Could you check a few things on this model? Use its own coordinates, in mm. A direction names the side the tool comes from. Coordinates: 2 decimals unless noted, no trailing zeros. Order: outer loops, then holes, each group sorted by start corner. A loop starts at its lowest first (then second) coordinate and runs counter-clockwise, first axis right, second up. Notation, with made-up numbers: (21.25, 50) - (35.25, 50) arc R26 cw to (35.25, 78) - close; hole circle Ø2 at (-3, 81.5). An arc over 180 degrees is marked (long way). One line per item, written item: value.
from build123d import *

# Parameters (mm, degrees)
SKETCH1_R           = 1.1
BOSS_EXTRUDE1_DEPTH = 5
SKETCH4_W           = 14
SKETCH4_H           = 12
BOSS_EXTRUDE3_DEPTH = 9
SKETCH5_W           = 10
SKETCH5_H           = 6
CUT_EXTRUDE2_DEPTH  = 9
CUT_EXTRUDE3_START  = 5
SKETCH7_R           = 1.1
CUT_EXTRUDE3_DEPTH  = 15
FILLET1_R           = 5
FILLET2_R           = 5


with BuildPart() as part:
    # Sketch1 → Boss-Extrude1 (new body)
    with BuildSketch(Plane.XY):
        with BuildLine():
            ThreePointArc((0, 3.5), (-3.5, 0), (0, -3.5))
            Line((0, -3.5), (83.5, -3.5))
            ThreePointArc((83.5, -3.5), (87, 0), (83.5, 3.5))
            Line((83.5, 3.5), (0, 3.5))
        make_face()
        Circle(SKETCH1_R, mode=Mode.SUBTRACT)
        with Locations((83.5, 0)):
            Circle(SKETCH1_R, mode=Mode.SUBTRACT)
    extrude(amount=BOSS_EXTRUDE1_DEPTH)

    # Sketch4 → Boss-Extrude3 (add)
    with BuildSketch(Plane(origin=(0, 3.5, 0), x_dir=(1, 0, 0), z_dir=(0, 1, 0))):
        with Locations((3, -2.5)):
            Rectangle(SKETCH4_W, SKETCH4_H)
    extrude(amount=-BOSS_EXTRUDE3_DEPTH)

    # Sketch5 → Cut-Extrude2 (cut)
    with BuildSketch(Plane.XZ.offset(5.5)):
        with Locations((1, 2.5)):
            Rectangle(SKETCH5_W, SKETCH5_H)
    extrude(amount=-CUT_EXTRUDE2_DEPTH, mode=Mode.SUBTRACT)

    # Sketch7 → Cut-Extrude3 (cut)
    with BuildSketch(Plane(origin=(0, 0, 0), x_dir=(-1, 0, 0), z_dir=(0, 0, -1)).offset(CUT_EXTRUDE3_START)):
        with Locations((0.5, 0)):
            Circle(SKETCH7_R)
    extrude(amount=-CUT_EXTRUDE3_DEPTH, mode=Mode.SUBTRACT)

    # Fillet1
    # the kernel refuses this fillet: 5 mm, written as the material it adds along each edge
    with BuildSketch(Plane(origin=(10, 3.5, 5), x_dir=(0, 0, 1), z_dir=(0, -1, 0))) as fillet1_piece_1:
        with BuildLine():
            CenterArc((5, -4.769696007), FILLET1_R, 107.457603124, 72.542396876)
            Line((0, -4.769696007), (-0.1, -4.769696007))
            Line((-0.1, -4.769696007), (-0.1, 0))
            Line((-0.1, 0), (0, 0.1))
            ThreePointArc((0, 0.1), (1.75, 0.1), (3.47, 0.09539392))
            Line((3.47, 0.09539392), (3.5, 0))
        make_face()
    extrude(amount=7)
    with BuildSketch(Plane(origin=(10, 3.5, 0), x_dir=(1, 0, 0), z_dir=(0, -1, 0))) as fillet1_piece_2:
        with BuildLine():
            CenterArc((4.769696007, -5), FILLET1_R, 90, 72.542396876)
            Line((0, -3.5), (-0.09539392, -3.47))
            ThreePointArc((-0.09539392, -3.47), (-0.1, -1.75), (-0.1, 0))
            Line((-0.1, 0), (0, 0.1))
            Line((0, 0.1), (4.769696007, 0.1))
            Line((4.769696007, 0.1), (4.769696007, 0))
        make_face()
    extrude(amount=7)

    # Fillet2
    fillet2_edges = [part.edges().sort_by_distance(p)[0] for p in [
        (6, 3.5, 2.5),
    ]]
    fillet(fillet2_edges, radius=FILLET2_R)


solid = part.part
Item 1: For faces 5 (the face through (7.43, 2, 2.54)), 6 (the face through (6, -4, 2)), 7 (the face through (50, 0, 5)), 8 (the face through (50, 0, 0)), 9 (the face through (10, -4, 3)), which set-ups out of +Z, -Z, +X, -X, +Y, -Y let a thin tool reach every point of the face, with its end or its side?
Conclusion:
face 5: -X, +Y
face 6: -X, +Y, -Y
face 7: +Z, +X, +Y, -Y
face 8: -Z, +X, +Y, -Y
face 9: +Z, -Z, +X, -Y
Item 2: If I drill on probe 1 along Y at (x, z) = (83.5, 1.85); probe 2 along Y at (x, z) = (-0.5, 7.15); probe 3 along Z at (x, y) = (1, -0.25), over which ranges is the centre line in solid material (lowest first)?
Conclusion:
probe 1: -3.5 to -1.1, 1.1 to 3.5
probe 2: -5.5 to -1.1, 1.1 to 3.5
probe 3: -3.5 to -0.5, 5.5 to 8.5
Item 3: I want a section at B-B on y = 0. Please give me the cut outline in (x, z), then the cut area to 3 significant figures.
Conclusion:
outline: (-4, -3.5) - (-1.6, -3.5) - (-1.6, -0.5) - (-4, -0.5) - close; (-4, 5.5) - (-1.6, 5.5) - (-1.6, 8.5) - (-4, 8.5) - close; (0.6, -3.5) - (10, -3.5) arc R5 cw to (14.77, 0) - (82.4, 0) - (82.4, 5) - (14.77, 5) arc R5 cw to (10, 8.5) - (0.6, 8.5) - (0.6, 5.5) - (6.23, 5.5) - (6.23, -0.5) - (0.6, -0.5) - close; (84.6, 0) - (87, 0) - (87, 5) - (84.6, 5) - close
area: 476 mm²
Item 4: I want a section at D-D on x = 69.5. Please give me the cut outline in (y, z).
Conclusion:
outline: (-3.5, 0) - (3.5, 0) - (3.5, 5) - (-3.5, 5) - close
Item 5: I want a section at C-C on z = 4. Please give me the cut outline in (x, y), then the cut area to 3 significant figures.
Conclusion:
outline: (6, -5.5) - (10, -5.5) - (10, -3.5) - (83.5, -3.5) arc R3.5 ccw to (83.5, 3.5) - (11, 3.5) arc R5 ccw to (6, -1.5) - close; hole circle Ø2.2 at (83.5, 0)
area: 561 mm²
Item 6: I want a section at A-A on x = -0.5. Please give me the cut outline in (y, z).
Conclusion:
outline: (-5.5, -3.5) - (-1.1, -3.5) - (-1.1, -0.5) - (-5.5, -0.5) - close; (-5.5, 5.5) - (-1.1, 5.5) - (-1.1, 8.5) - (-5.5, 8.5) - close; (1.1, -3.5) - (3.5, -3.5) - (3.5, -0.5) - (1.1, -0.5) - close; (1.1, 5.5) - (3.5, 5.5) - (3.5, 8.5) - (1.1, 8.5) - close
Item 7: Thinking about a two-plate mould opening in X: for faces 1 (the face through (-4, -1, -2)), 2 (the face through (11.85, 0.05, -0.94)), 3 (the face through (82.4, 0, 2.5)), 4 (the face through (-1.55, 0.33, -2.02)), which applies, pulls with the +X half, pulls with the -X half, needs draft (parallel to the pull), parting line crosses it, or undercut?
Conclusion:
face 1: pulls with the -X half
face 2: pulls with the +X half
face 3: undercut
face 4: undercut
Item 8: I'm going to push flat-ended pins straight in: pin 1 Ø0.6 at (y, z) = (-5, 2) entering from +X; pin 2 Ø4 at (x, y) = (26.5, -1) entering from +Z; pin 3 Ø1 at (x, y) = (18, -1) entering from -Z. Where does each tip first touch, or does it pass through?
Conclusion:
pin 1: x = 10
pin 2: z = 5
pin 3: z = 0
